Here's how the part is built. I have some questions about the finished solid (model axes, mm). Face numbers are marked on the shaded views. A direction names the side the tool comes from. Give positions to 0.01 mm unless a question says otherwise; leave off trailing zeros. Loops run counter-clockwise (first coordinate to the right, second up) from the corner with the lowest first, then second, coordinate; pieces in that order, holes last. Notation, with made-up numbers: (38, -39) -> (64, -39) arc R25 ccw to (64, -8) -> close; hole circle Ø1 at (80.5, 47). An arc over 180 degrees is marked (long way). Answer in a Markdown table with one row per item. Add a question column.
Item 1: If we section it at A-A (y = 5.75): Write out the boundary of the cut face in (x, z).
Item 2: For P1, Ø2, axis at x = -1.5, y = 3, coming from the +Z side; P2, Ø1.5, axis at x = 0, y = 4.5, coming from the -Z side; P3, Ø2, axis at x = 2, y = 8.5, coming from the +Z side, each with a flat end and sliding along its axis, tell me the tip position at first contact or that it passes through.
Item 3: If we section it at D-D (x = -1.15): Write out the boundary of the cut face in (y, z), then the cut area to 3 significant figures.
Item 4: If we section it at B-B (x = 1.75): Write out the boundary of the cut face in (y, z), then the cut area to 3 significant figures.
Item 5: If we section it at C-C (z = 0.55): Write out the boundary of the cut face in (x, y).
Item 6: Which directions (+Z, -Z, +X, -X, +Y, -Y) give clear straight access to the entire face, cutting with the end or side of a thin tool? Please do the marked faces 1, 2, 3, 4 and 5.
Item 7: If I drill on line 1 (Y direction, x = -2.4, z = -1.1); line 2 (Z direction, x = 0.4, y = 5.5), over which ranges is the centre line in solid material (lowest first)?
```python
from build123d import *

# Parameters (mm, degrees)
SKETCH1_W           = 6
SKETCH1_H           = 6
BOSS_EXTRUDE1_DEPTH = 1
FILLET1_R           = 1
SKETCH2_W           = 2.9
SKETCH2_H           = 2.9
BOSS_EXTRUDE2_DEPTH = 9
FILLET2_R           = 0.5
FILLET3_R           = 0.5
CHAMFER1_SIZE       = 0.5


with BuildPart() as part:
    # Sketch1 → Boss-Extrude1 (new body)
    with BuildSketch(Plane(origin=(0, 0, 0), x_dir=(1, 0, 0), z_dir=(0, 1, 0))):
        Rectangle(SKETCH1_W, SKETCH1_H)
    extrude(amount=BOSS_EXTRUDE1_DEPTH)

    # Fillet1
    fillet1_edges = [part.edges().sort_by_distance(p)[0] for p in [
        (3, 0.5, 3),
        (-3, 0.5, 3),
        (-3, 0.5, -3),
        (3, 0.5, -3),
    ]]
    fillet(fillet1_edges, radius=FILLET1_R)

    # Sketch2 → Boss-Extrude2 (add)
    with BuildSketch(Plane(origin=(0, 1, 0), x_dir=(1, 0, 0), z_dir=(0, 1, 0))):
        Rectangle(SKETCH2_W, SKETCH2_H)
    extrude(amount=BOSS_EXTRUDE2_DEPTH)

    # Fillet2
    fillet2_edges = [part.edges().sort_by_distance(p)[0] for p in [
        (1.45, 5.5, 1.45),
        (1.45, 5.5, -1.45),
        (-1.45, 5.5, -1.45),
        (-1.45, 5.5, 1.45),
    ]]
    fillet(fillet2_edges, radius=FILLET2_R)

    # Fillet3
    fillet3_edges = [part.edges().sort_by_distance(p)[0] for p in [
        (0, 10, -1.45),
        (1.45, 10, 0),
        (-1.45, 10, 0),
        (0, 10, 1.45),
        (-1.303553391, 10, 1.303553391),
        (1.303553391, 10, 1.303553391),
        (-1.303553391, 10, -1.303553391),
        (1.303553391, 10, -1.303553391),
    ]]
    fillet(fillet3_edges, radius=FILLET3_R)

    # Chamfer1
    chamfer1_edges = [part.edges().sort_by_distance(p)[0] for p in [
        (0, 0, 3),
        (3, 0, 0),
        (-3, 0, 0),
        (0, 0, -3),
        (2.707106781, 0, 2.707106781),
        (2.707106781, 0, -2.707106781),
        (-2.707106781, 0, -2.707106781),
        (-2.707106781, 0, 2.707106781),
    ]]
    chamfer(chamfer1_edges, length=CHAMFER1_SIZE)


solid = part.part
```
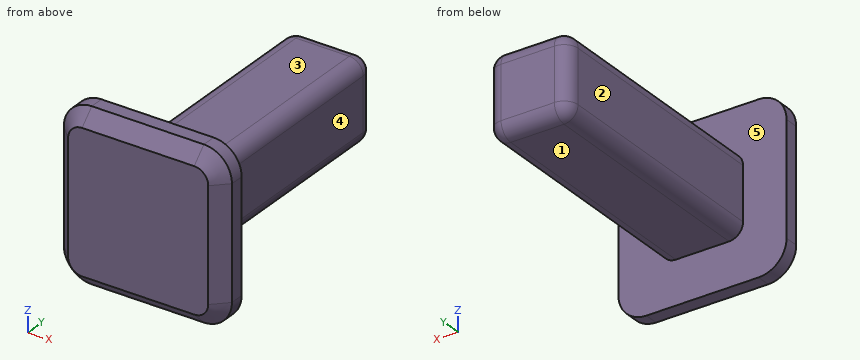
Recorded:
| question | item | result |
|---|---|---|
| 1 | outline | (-1.45, -0.95) arc R0.5 ccw to (-0.95, -1.45) -> (0.95, -1.45) arc R0.5 ccw to (1.45, -0.95) -> (1.45, 0.95) arc R0.5 ccw to (0.95, 1.45) -> (-0.95, 1.45) arc R0.5 ccw to (-1.45, 0.95) -> close |
| 2 | P1 | stops at z = 1.45 |
| 2 | P2 | stops at z = -1.45 |
| 2 | P3 | stops at z = 1.45 |
| 3 | outline | (0, -2.5) -> (0.5, -3) -> (1, -3) -> (1, -1.41) -> (9.5, -1.41) arc R0.46 ccw to (9.96, -0.95) -> (9.96, 0.95) arc R0.46 ccw to (9.5, 1.41) -> (1, 1.41) -> (1, 3) -> (0.5, 3) -> (0, 2.5) -> close |
| 3 | area | 30.9 mm^2 |
| 4 | outline | (0, -2.5) -> (0.5, -3) -> (1, -3) -> (1, 3) -> (0.5, 3) -> (0, 2.5) -> close |
| 4 | area | 5.75 mm^2 |
| 5 | outline | (-3, 0.5) -> (-2.5, 0) -> (2.5, 0) -> (3, 0.5) -> (3, 1) -> (1.45, 1) -> (1.45, 9.5) arc R0.5 ccw to (0.95, 10) -> (-0.95, 10) arc R0.5 ccw to (-1.45, 9.5) -> (-1.45, 1) -> (-3, 1) -> close |
| 6 | face 1 | -Z, +X, -X, +Y |
| 6 | face 2 | +Z, -Z, -X, +Y |
| 6 | face 3 | +Z, +X, -X, +Y |
| 6 | face 4 | +Z, -Z, +X, +Y |
| 6 | face 5 | +Y |
| 7 | line 1 | y = 0 to 1 |
| 7 | line 2 | z = -1.45 to 1.45 |
